```python
from build123d import *

# Parameters (mm, degrees)
SKETCH_1_R      = 2
SKETCH_1_R_2    = 1
EXTRUDE_1_DEPTH = 2


with BuildPart() as part:
    # 草图1 → 凸台-拉伸1 (new body)
    with BuildSketch(Plane.XY):
        with BuildLine():
            Line((-22.340449028, 112.565520938), (-22.340449028, 35.565520938))
            Line((-22.340449028, 35.565520938), (-41.340449028, 35.565520938))
            Line((-41.340449028, 35.565520938), (-41.340449028, 19.565520938))
            Line((-41.340449028, 19.565520938), (14.659550972, 19.565520938))
            Line((14.659550972, 19.565520938), (14.659550972, 35.565520938))
            Line((14.659550972, 35.565520938), (-4.340449028, 35.565520938))
            Line((-4.340449028, 35.565520938), (-4.340449028, 112.565520938))
            ThreePointArc((-4.340449028, 112.565520938), (-13.340449028, 121.565520938), (-22.340449028, 112.565520938))
        make_face()
        with Locations((-33.340449028, 27.565520938)):
            Circle(SKETCH_1_R, mode=Mode.SUBTRACT)
        with Locations(Location((6.659550972, 27.565520938, 0), (0, 0, 180))):
            Circle(SKETCH_1_R, mode=Mode.SUBTRACT)
        with Locations((-7.340449028, 112.565520938)):
            Circle(SKETCH_1_R_2, mode=Mode.SUBTRACT)
        with Locations(Location((-19.340449028, 112.565520938, 0), (0, 0, 180))):
            Circle(SKETCH_1_R_2, mode=Mode.SUBTRACT)
        with Locations((-13.340449028, 47.565520938)):
            Circle(SKETCH_1_R, mode=Mode.SUBTRACT)
    extrude(amount=EXTRUDE_1_DEPTH)


solid = part.part
```
Part model, mm, in its own coordinate system. A direction names the side the tool comes from. Round coordinates to 2 decimals unless told otherwise and drop trailing zeros. Loops run counter-clockwise (first coordinate to the right, second up) from the corner with the lowest first, then second, coordinate; pieces in that order, holes last.
1. Slice it at D-D (y = 86.5). Give the cut face in (x, z).
Solutions:
outline: (-22.34, 0) - (-4.34, 0) - (-4.34, 2) - (-22.34, 2) - close
2. Flat gauge pins, fed straight in: pin 1 (3 mm diameter, centred on x = -33.34, y = 27.57, fed in from -Z); pin 2 (1 mm diameter, centred on y = 93, z = 1.5, fed in from +X); pin 3 (0.6 mm diameter, centred on y = 69.5, z = 1, fed in from -X). Where does each tip first touch, or does it go through?
Solutions:
pin 1: passes through
pin 2: stops at x = -4.34
pin 3: stops at x = -22.34
3. Slice it at B-B (x = -33). Give the cut face in (y, z), and give its area (3 significant figures).
Solutions:
outline: (19.57, 0) - (25.59, 0) - (25.59, 2) - (19.57, 2) - close; (29.54, 0) - (35.57, 0) - (35.57, 2) - (29.54, 2) - close
area: 24.1 mm2
4. 3-axis set-ups, long thin cutter, end or side, ignore diameter. For faces 4 (the face through (-13.6, 49.55, 0.99)), 5 (the face through (-32, 35.566, 1)), 6 (the face through (5, 35.566, 1)): which of +Z, -Z, +X, -X, +Y, -Y reach the whole face in a straight line?
Solutions:
face 4: +Z, -Z
face 5: +Z, -Z, -X, +Y
face 6: +Z, -Z, +X, +Y
5. Slice it at A-A (z = 1.3). Give the cut face in (x, y), and give its area (3 significant figures).
Solutions:
outline: (-41.34, 19.57) - (14.66, 19.57) - (14.66, 35.57) - (-4.34, 35.57) - (-4.34, 112.57) arc R9 ccw to (-22.34, 112.57) - (-22.34, 35.57) - (-41.34, 35.57) - close; hole circle Ø4 at (-33.34, 27.57); hole circle Ø2 at (-19.34, 112.57); hole circle Ø4 at (-13.34, 47.57); hole circle Ø2 at (-7.34, 112.57); hole circle Ø4 at (6.66, 27.57)
area: 2,370 mm2
6. Slice it at C-C (x = -3). Give the cut face in (y, z), and give its area (3 significant figures).
Solutions:
outline: (19.57, 0) - (35.57, 0) - (35.57, 2) - (19.57, 2) - close
area: 32.0 mm2
7. Drill centre lines: line 1 along X through (y, z) = (29, 0.4); line 2 along X through (y, z) = (100.5, 1.8); line 3 along Y through (x, z) = (-23, 1.3). Where is each one in solid material? Low to high.
Solutions:
line 1: x = -41.34 to -34.73, -31.95 to 5.27, 8.05 to 14.66
line 2: x = -22.34 to -4.34
line 3: y = 19.57 to 35.57
8. Two-plate mould, pull along X, no slides. Class faces 1 (the face through (-14, 60, 2)), 2 (the face through (5.74, 29.34, 0.99)), 3 (the face through (-41.34, 28, 1)): pulls with the +X half, pulls with the -X half, needs draft (parallel to the pull), parting line crosses it, or undercut.
Solutions:
face 1: needs draft
face 2: undercut
face 3: pulls with the -X half
